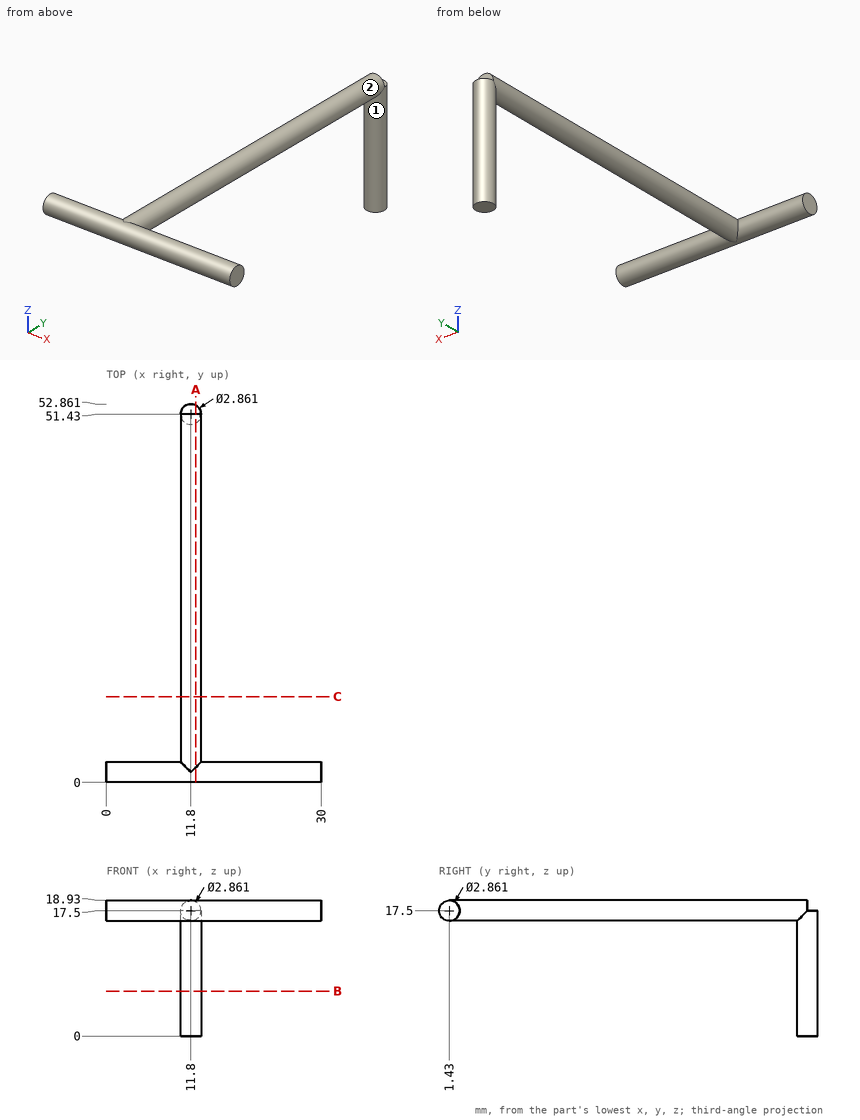
Answer from the drawing. Dimensions are ordinates in mm from the lowest x, y and z of the part. A direction names the side the tool comes from. Round coordinates to 2 decimals unless told otherwise and drop trailing zeros. Write each loop counter-clockwise with the first axis right and the second up, starting at its lowest first coordinate (ties: lowest second). Pieces come first, ordered by that corner, then holes.
1. The part is cut by section A-A, the plane x = 12.5. Determine the outline of the cut face in (y, z).
2. Straight lines are drawn through the part: L1, parallel to X at y = 50.5, z = 4 (1 decimal); L2, parallel to Y at x = 9, z = 17. For each, find the intervals that lie inside material, in ascending order.
3. Given pin 1 Ø5 at (x, y) = (11, 19.5) entering from -Z; pin 2 Ø4 at (x, z) = (12, 8.5) entering from -Y; pin 3 Ø3 at (x, z) = (9, 16) entering from -Y; pin 4 Ø3 at (y, z) = (14.5, 15.5) entering from +X, each flat-ended and moving along its own axis, determine where each tip first touches the part or whether it passes through.
4. Which of the six approach directions +Z, -Z, +X, -X, +Y, -Y give full straight-line access (tool end or side, diameter ignored) to the marked faces 1 and 2?
5. The part is cut by section B-B, the plane z = 6.25. Determine the outline of the cut face in (x, y).
6. The part is cut by section C-C, the plane y = 12. Determine the outline of the cut face in (x, z).
Values:
1. outline: (2.13, 16.25) - (50.18, 16.25) - (50.18, 0) - (52.68, 0) - (52.68, 17.5) - (51.43, 17.5) - (51.43, 18.75) - (2.13, 18.75) arc R1.43 ccw (long way) to start
2. L1: x = 10.7 to 12.9
2. L2: y = 0.09 to 2.77
3. pin 1: stops at z = 16.07
3. pin 2: stops at y = 50
3. pin 3: stops at y = 0
3. pin 4: stops at x = 13.14
4. face 1: -Z
4. face 2: none
5. outline: circle Ø2.86 at (11.8, 51.43)
6. outline: circle Ø2.86 at (11.8, 17.5)
